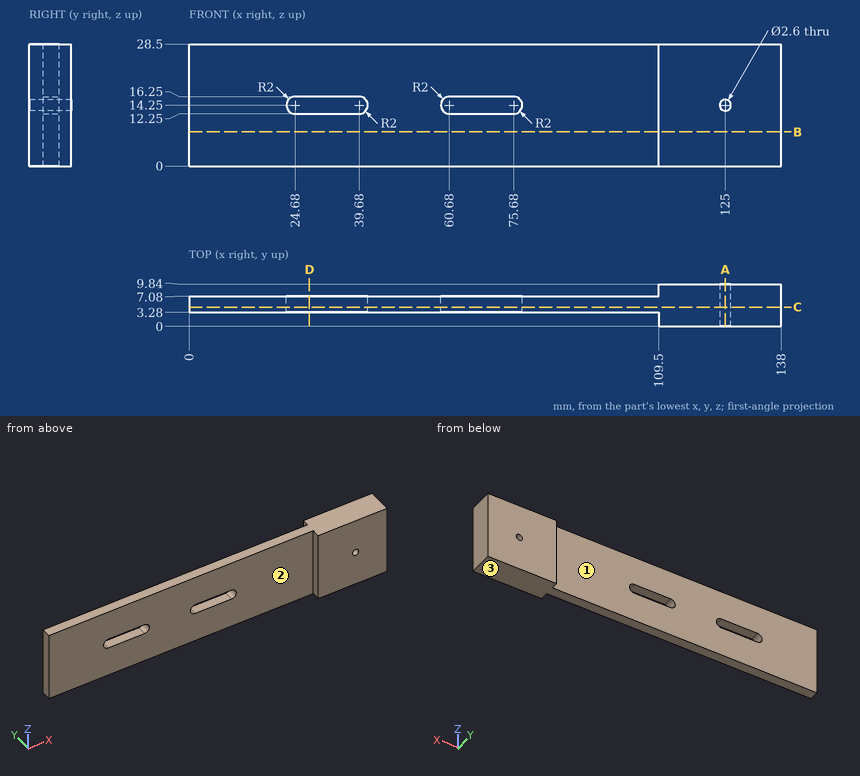
Part print with two shaded views. Sizes in mm from the minimum x, y, z corner. A direction names the side the tool comes from. Give positions to 0.01 mm unless a question says otherwise; leave off trailing zeros. Loops run counter-clockwise (first coordinate to the right, second up) from the corner with the lowest first, then second, coordinate; pieces in that order, holes last. Notation, with made-up numbers: (66, -2) - (77, -2) arc R3 ccw to (77, 3) - close; hole circle Ø9 at (33, -35.5). An arc over 180 degrees is marked (long way). Put each result on its own line as item: value.
Q1. Flat gauge pins, fed straight in: pin 1 (2.5 mm diameter, centred on y = 1, z = 12.5, fed in from -X); pin 2 (3 mm diameter, centred on x = 29.5, z = 25, fed in from -Y); pin 3 (8 mm diameter, centred on x = 69, z = 23, fed in from +Y). Where does each tip first touch, or does it go through?
Filled in:
pin 1: stops at x = 109.5
pin 2: stops at y = 3.28
pin 3: stops at y = 7.08
Q2. Slice it at A-A (x = 125). Give the cut face in (y, z), plus the area to 3 significant figures.
Filled in:
outline: (0, 0) - (9.84, 0) - (9.84, 12.95) - (0, 12.95) - close; (0, 15.55) - (9.84, 15.55) - (9.84, 28.5) - (0, 28.5) - close
area: 255 mm²
Q3. Tool access for the marked faces 1, 2 and 3: list every direction of +Z, -Z, +X, -X, +Y, -Y with a clear straight run to the whole face (end or side of a thin tool).
Filled in:
face 1: +Z, -Z, -X, +Y
face 2: +Z, -Z, -X, -Y
face 3: -Z, +X, -X, +Y, -Y
Q4. Slice it at C-C (y = 4.5). Give the cut face in (x, z), plus the area to 3 significant figures.
Filled in:
outline: (0, 0) - (138, 0) - (138, 28.5) - (0, 28.5) - close; hole (22.68, 14.25) arc R2 ccw to (24.68, 12.25) - (39.68, 12.25) arc R2 ccw to (41.68, 14.25) arc R2 ccw to (39.68, 16.25) - (24.68, 16.25) arc R2 ccw to start; hole (58.68, 14.25) arc R2 ccw to (60.68, 12.25) - (75.68, 12.25) arc R2 ccw to (77.68, 14.25) arc R2 ccw to (75.68, 16.25) - (60.68, 16.25) arc R2 ccw to start; hole circle Ø2.6 at (125, 14.25)
area: 3,780 mm²
Q5. Slice it at B-B (z = 8). Give the cut face in (x, y).
Filled in:
outline: (0, 3.28) - (109.5, 3.28) - (109.5, 0) - (138, 0) - (138, 9.84) - (109.5, 9.84) - (109.5, 7.08) - (0, 7.08) - close
Q6. Probe line 1 along Z through (x, y) = (125, 4); line 2 along Y through (x, z) = (8.5, 21.25); line 3 along X through (y, z) = (8.75, 14). List the from-to ranges inside material, lowest first.
Filled in:
line 1: z = 0 to 12.95, 15.55 to 28.5
line 2: y = 3.28 to 7.08
line 3: x = 109.5 to 123.72, 126.28 to 138
Q7. Slice it at D-D (x = 28). Give the cut face in (y, z), plus the area to 3 significant figures.
Filled in:
outline: (3.28, 0) - (7.08, 0) - (7.08, 12.25) - (3.28, 12.25) - close; (3.28, 16.25) - (7.08, 16.25) - (7.08, 28.5) - (3.28, 28.5) - close
area: 93.1 mm²
